```python
from build123d import *

# Parameters (mm, degrees)
CYLINDER022_R     = 2.2
CYLINDER022_DEPTH = 0.5
CYLINDER021_R     = 3.15
CYLINDER021_DEPTH = 0.5


with BuildPart() as cylinder022:
    # Cylinder022 → Cylinder022 (new body)
    with BuildSketch(Plane.XY):
        Circle(CYLINDER022_R)
    extrude(amount=CYLINDER022_DEPTH)


with BuildPart() as f_0p5_spacer:
    # Cylinder021 → Cylinder021 (new body)
    with BuildSketch(Plane.XY):
        Circle(CYLINDER021_R)
    extrude(amount=CYLINDER021_DEPTH)

    # Cut001021: cut Cylinder022
    add(cylinder022.part, mode=Mode.SUBTRACT)


solid = f_0p5_spacer.part
```
The listing builds one solid part. Answer for the finished solid, in the listing's coordinates (mm). Coordinates: 2 decimals unless noted, no trailing zeros. Write each loop counter-clockwise with the first axis right and the second up, starting at its lowest first coordinate (ties: lowest second). Pieces come first, ordered by that corner, then holes. Notation, with made-up numbers: (-13.5, 57) - (21.5, 57) arc R8 ccw to (21.5, 65) - close; hole circle Ø4 at (-21, 23). An arc over 180 degrees is marked (long way). Return JSON: item names as keys, results as strings. Group by question number.
1. Straight lines are drawn through the part: L1, parallel to Y at x = 0, z = 0.25; L2, parallel to X at y = -2, z = 0.1; L3, parallel to Y at x = 1.25, z = 0.1. For each, find the intervals that lie inside material, in ascending order.
2. A cutting plane is placed at C-C, the plane z = 0.3. Determine the outline of the cut face in (x, y), plus the area to 3 significant figures.
3. A cutting plane is placed at A-A, the plane x = 0. Determine the outline of the cut face in (y, z).
4. Determine the mould class of faces 1 (the cylindrical face through (2.1, 0.66, 0.25)), 2 (the cylindrical face through (-2.5, -1.917, 0.246)), 3 (the flat face through (1.4, -2.1, 0.5)) for opening direction X: released by +X, released by -X, zero draft, split by the parting line, or undercut.
Ans:
{
 "1": {"L1": "-3.15 to -2.2, 2.2 to 3.15", "L2": "-2.43 to -0.92, 0.92 to 2.43", "L3": "-2.89 to -1.81, 1.81 to 2.89"},
 "2": {"outline": "circle Ø6.3 at (0, 0); hole circle Ø4.4 at (0, 0)", "area": "16.0 mm²"},
 "3": {"outline": "(-3.15, 0) - (-2.2, 0) - (-2.2, 0.5) - (-3.15, 0.5) - close; (2.2, 0) - (3.15, 0) - (3.15, 0.5) - (2.2, 0.5) - close"},
 "4": {"face 1": "undercut", "face 2": "split by the parting line", "face 3": "zero draft"}
}
